CAD build for the part. Positions are in the model's coordinates, mm. Give positions to 0.01 mm unless a question says otherwise; leave off trailing zeros. Order: outer loops, then holes, each group sorted by start corner. A loop starts at its lowest first (then second) coordinate and runs counter-clockwise, first axis right, second up.
from build123d import *

# Parameters (mm, degrees)
F0_R     = 19.05
F0_R_2   = 76.2
F1_DEPTH = 16.51
F2_SIZE  = 5.08
F3_SIZE  = 5.08
F4_SIZE  = 3.175
F5_R     = 6.35


with BuildPart() as f1:
    # F0 (on Front) → F1 (new body)
    with BuildSketch(Plane.XZ):
        with BuildLine():
            Line((95.25, 101.6), (-95.25, 101.6))
            ThreePointArc((-95.25, 101.6), (-117.70064, 92.30064), (-127, 69.85))
            Line((-127, 69.85), (-127, -69.85))
            ThreePointArc((-127, -69.85), (-117.70064, -92.30064), (-95.25, -101.6))
            Line((-95.25, -101.6), (95.25, -101.6))
            ThreePointArc((95.25, -101.6), (117.70064, -92.30064), (127, -69.85))
            Line((127, -69.85), (127, 69.85))
            ThreePointArc((127, 69.85), (117.70064, 92.30064), (95.25, 101.6))
        make_face()
        with Locations((-88.9, -63.5)):
            Circle(F0_R, mode=Mode.SUBTRACT)
        with Locations((88.9, -63.5)):
            Circle(F0_R, mode=Mode.SUBTRACT)
        Circle(F0_R_2, mode=Mode.SUBTRACT)
        with Locations((-88.9, 63.5)):
            Circle(F0_R, mode=Mode.SUBTRACT)
        with Locations((88.9, 63.5)):
            Circle(F0_R, mode=Mode.SUBTRACT)
    extrude(amount=F1_DEPTH)

    # F2
    f2_edges = [f1.edges().sort_by_distance(p)[0] for p in [
        (0, -16.51, 101.6),
        (-117.70064, -16.51, 92.30064),
    ]]
    chamfer(f2_edges, length=F2_SIZE)

    # F3
    f3_edges = [f1.edges().sort_by_distance(p)[0] for p in [
        (127, 0, 0),
    ]]
    chamfer(f3_edges, length=F3_SIZE)

    # F4
    f4_edges = [f1.edges().sort_by_distance(p)[0] for p in [
        (-107.95, -16.51, 63.5),
        (69.85, -16.51, 63.5),
        (69.85, -16.51, -63.5),
        (-107.95, -16.51, -63.5),
        (-107.95, 0, 63.5),
        (69.85, 0, 63.5),
        (69.85, 0, -63.5),
        (-107.95, 0, -63.5),
    ]]
    chamfer(f4_edges, length=F4_SIZE)

    # F5
    f5_edges = [f1.edges().sort_by_distance(p)[0] for p in [
        (-76.2, 0, 0),
        (-76.2, -16.51, 0),
    ]]
    fillet(f5_edges, radius=F5_R)


solid = f1.part
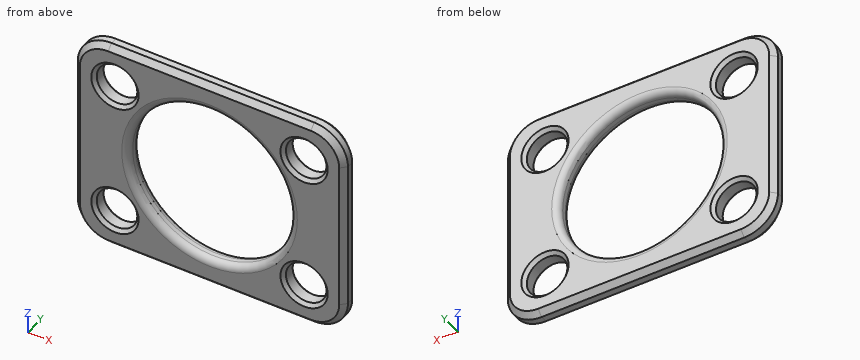
1. Saw through at C-C on z = 63.5. State how many separate pieces and enclosed holes the cut face has, plus the area to 3 significant figures.
2. Saw through at A-A on z = 0. Give the cut face in (x, y), plus the area to 3 significant figures.
3. Pin check, flat tips, straight feed: P1, Ø5, axis at y = -1.5, z = -74.5, coming from the +X side; P2, Ø8, axis at y = -6.5, z = -78, coming from the +X side. Stop position of each tip, or through.
4. Saw through at B-B on x = 88.9. Give the cut face in (y, z) (3 decimals).
5. Wall check: line 1 (Z direction, x = 88.9, y = -8.5); line 2 (X direction, y = -13, z = 61); line 3 (Z direction, x = 0, y = -8.1). Give the ranges that are in metal, low to high.
Reported:
1. separate pieces: 4
1. enclosed holes: 0
1. area: 1,390 mm2
2. outline: (-127, -11.43) - (-121.92, -16.51) - (-82.55, -16.51) arc R6.35 ccw to (-76.2, -10.16) - (-76.2, -6.35) arc R6.35 ccw to (-82.55, 0) - (-121.92, 0) - (-127, -5.08) - close; (76.2, -10.16) arc R6.35 ccw to (82.55, -16.51) - (121.92, -16.51) - (127, -11.43) - (127, -5.08) - (121.92, 0) - (82.55, 0) arc R6.35 ccw to (76.2, -6.35) - close
2. area: 1,590 mm2
3. P1: stops at x = 125.59
3. P2: stops at x = 126.73
4. outline: (-16.51, -96.52) - (-11.43, -101.6) - (-5.08, -101.6) - (0, -96.52) - (0, -85.725) - (-3.175, -82.55) - (-13.335, -82.55) - (-16.51, -85.725) - close; (-16.51, -41.275) - (-13.335, -44.45) - (-3.175, -44.45) - (0, -41.275) - (0, 41.275) - (-3.175, 44.45) - (-13.335, 44.45) - (-16.51, 41.275) - close; (-16.51, 85.725) - (-13.335, 82.55) - (-3.175, 82.55) - (0, 85.725) - (0, 96.52) - (-5.08, 101.6) - (-11.43, 101.6) - (-16.51, 96.52) - close
5. line 1: z = -101.6 to -82.55, -44.45 to 44.45, 82.55 to 101.6
5. line 2: x = -125.43 to -107.79, -70.01 to -46.78, 46.78 to 70.01, 107.79 to 125.43
5. line 3: z = -101.6 to -76.2, 76.2 to 101.6
